Can you work these out from the model? Positions are in its coordinate system, mm. Give positions to 0.01 mm unless a question says otherwise; leave off trailing zeros. Order: outer loops, then holes, each group sorted by start corner. A loop starts at its lowest first (then second) coordinate and runs counter-clockwise, first axis right, second up. Notation, with made-up numbers: (-25, -31) -> (2, -31) arc R30 cw to (2, 1) -> close; hole circle Ø5 at (65, 38). An arc over 180 degrees is marked (long way). Answer as a JSON object with one key per item and string values.
```python
from build123d import *

# Parameters (mm, degrees)
SKETCH1_W                    = 76
SKETCH1_H                    = 85
BOSS_EXTRUDE1_DEPTH          = 3
M2_5_CLEARANCE_HOLE1_D       = 2.7
CSK_FOR_M3_SFHCS1_AT_2_COUNT = 2
CSK_FOR_M3_SFHCS1_AT_2_PITCH = 31.5
CSK_FOR_M3_SFHCS1_AT_3_COUNT = 2
CSK_FOR_M3_SFHCS1_AT_3_PITCH = 73.131730459
CSK_FOR_M3_SFHCS1_AT_4_COUNT = 2
CSK_FOR_M3_SFHCS1_AT_4_PITCH = 66
FILLET1_R                    = 3


with BuildPart() as part:
    # Sketch1 → Boss-Extrude1 (new body)
    with BuildSketch(Plane(origin=(0, 0, 0), x_dir=(1, 0, 0), z_dir=(0, 1, 0))):
        Rectangle(SKETCH1_W, SKETCH1_H)
    extrude(amount=BOSS_EXTRUDE1_DEPTH)

    # M2.5 Clearance Hole1 (through all)
    with Locations(Plane(origin=(0, 3, 0), x_dir=(1, 0, 0), z_dir=(0, 1, 0))):
        with Locations((-24.5, 39), (-24.5, -19), (24.5, -19), (24.5, 39)):
            Hole(M2_5_CLEARANCE_HOLE1_D / 2)

    # Sketch5 → CSK for M3 SFHCS1 (revolve, cut)
    with BuildSketch(Plane(origin=(-33, 3, 24.5), x_dir=(0, 0, 1), z_dir=(1, 0, 0))):
        Polygon((0, 0), (0, 3), (1.6, 3), (1.6, 1.76), (3.36, 0), align=None)
    csk_for_m3_sfhcs1 = revolve(axis=Axis((-33, 9.35, 24.5), (0, -1, 0)), mode=Mode.SUBTRACT)

    # CSK for M3 SFHCS1 at 2: CSK for M3 SFHCS1 ×2
    with Locations(*[(0, 0, -i * CSK_FOR_M3_SFHCS1_AT_2_PITCH) for i in range(1, CSK_FOR_M3_SFHCS1_AT_2_COUNT)]):
        add(csk_for_m3_sfhcs1, mode=Mode.SUBTRACT)

    # CSK for M3 SFHCS1 at 3: CSK for M3 SFHCS1 ×2
    with Locations(*[Vector(0.9024810377836799, 0, -0.43072958621493834) * (i * CSK_FOR_M3_SFHCS1_AT_3_PITCH) for i in range(1, CSK_FOR_M3_SFHCS1_AT_3_COUNT)]):
        add(csk_for_m3_sfhcs1, mode=Mode.SUBTRACT)

    # CSK for M3 SFHCS1 at 4: CSK for M3 SFHCS1 ×2
    with Locations(*[(i * CSK_FOR_M3_SFHCS1_AT_4_PITCH, 0, 0) for i in range(1, CSK_FOR_M3_SFHCS1_AT_4_COUNT)]):
        add(csk_for_m3_sfhcs1, mode=Mode.SUBTRACT)

    # Fillet1
    fillet1_edges = [part.edges().sort_by_distance(p)[0] for p in [
        (-38, 1.5, -42.5),
        (38, 1.5, -42.5),
        (38, 1.5, 42.5),
        (-38, 1.5, 42.5),
    ]]
    fillet(fillet1_edges, radius=FILLET1_R)


solid = part.part
```
1. If we section it at C-C on x = -24.5: Please give me the cut outline in (y, z), then the cut area to 3 significant figures.
Worked answers:
{"outline": "(0, -42.5) -> (3, -42.5) -> (3, -40.35) -> (0, -40.35) -> close; (0, -37.65) -> (3, -37.65) -> (3, 17.65) -> (0, 17.65) -> close; (0, 20.35) -> (3, 20.35) -> (3, 42.5) -> (0, 42.5) -> close", "area": "239 mm²"}
2. If we section it at B-B on z = 24.5: Please give me the cut outline in (x, y).
Worked answers:
{"outline": "(-38, 0) -> (-34.6, 0) -> (-34.6, 1.24) -> (-36.36, 3) -> (-38, 3) -> close; (-31.4, 0) -> (31.4, 0) -> (31.4, 1.24) -> (29.64, 3) -> (-29.64, 3) -> (-31.4, 1.24) -> close; (34.6, 0) -> (38, 0) -> (38, 3) -> (36.36, 3) -> (34.6, 1.24) -> close"}
3. Please list where these lines run through material, in increasing order: L1, parallel to Z at x = -33, y = 0.35; L2, parallel to X at y = 0.95, z = 19; L3, parallel to X at y = 0.75, z = -7.
Worked answers:
{"L1": "-42.5 to -8.6, -5.4 to 22.9, 26.1 to 42.5", "L2": "-38 to -25.85, -23.15 to 23.15, 25.85 to 38", "L3": "-38 to -34.6, -31.4 to 31.4, 34.6 to 38"}
4. If we section it at A-A on x = 33: Please give me the cut outline in (y, z), then the cut area to 3 significant figures.
Worked answers:
{"outline": "(0, -42.5) -> (3, -42.5) -> (3, -10.36) -> (1.24, -8.6) -> (0, -8.6) -> close; (0, -5.4) -> (1.24, -5.4) -> (3, -3.64) -> (3, 21.14) -> (1.24, 22.9) -> (0, 22.9) -> close; (0, 26.1) -> (1.24, 26.1) -> (3, 27.86) -> (3, 42.5) -> (0, 42.5) -> close", "area": "230 mm²"}
5. Will these pins go through, and if not, where does the flat tip stop? pin 1 Ø5 at (x, z) = (33, -7) entering from +Y; pin 2 Ø4 at (x, z) = (-33, -7) entering from +Y.
Worked answers:
{"pin 1": "y = 2.14", "pin 2": "y = 1.64"}
6. If we mould it in two halves opening along Z, with no side actions, what happens to faces 1 (the face through (-25.747, 1.479, 19.517)), 2 (the face through (37.1, 1.52, 41.64)), 3 (the face through (-1, 3, -1))? For each: +Z half, -Z half, draft (parallel to the pull), parting line (faces both ways), or undercut.
Worked answers:
{"face 1": "undercut", "face 2": "+Z half", "face 3": "draft"}
